```python
from build123d import *

# Parameters (mm, degrees)
SKETCH_1_R          = 1.525
SKETCH_1_R_2        = 5
EXTRUDE_1_DEPTH     = 4
CUT_EXTRUDE_START   = -4
CUT_EXTRUDE_1_DEPTH = 4
FILLET_1_R          = 1


with BuildPart() as part:
    # 草图1 → 凸台-拉伸1 (new body)
    # profile 1 of 2: a face of its own
    with BuildSketch(Plane.XY):
        with BuildLine():
            ThreePointArc((12, 0), (7.073549415, 9.693549333), (-3.660816447, 11.427966702))
            ThreePointArc((-3.660816447, 11.427966702), (-10.576904144, -5.668253587), (7.48855525, -9.376648669))
            ThreePointArc((7.48855525, -9.376648669), (10.813479158, -5.202755856), (12, 0))
        make_face()
        with Locations((5.142300877, -6.128355545)):
            Circle(SKETCH_1_R, mode=Mode.SUBTRACT)
        with Locations((-6.128355545, -5.142300877)):
            Circle(SKETCH_1_R, mode=Mode.SUBTRACT)
        Circle(SKETCH_1_R_2, mode=Mode.SUBTRACT)
        with Locations((-5.142300877, 6.128355545)):
            Circle(SKETCH_1_R, mode=Mode.SUBTRACT)
        with Locations((6.128355545, 5.142300877)):
            Circle(SKETCH_1_R, mode=Mode.SUBTRACT)
    # profile 2 of 2: a face of its own
    with BuildSketch(Plane.XY):
        with BuildLine():
            Line((25.489995997, 5), (25.489995997, 15))
            Line((25.489995997, 15), (7.489995997, 15))
            Line((7.489995997, 15), (-3.660816447, 11.427966702))
            ThreePointArc((-3.660816447, 11.427966702), (7.073549415, 9.693549333), (12, 0))
            ThreePointArc((12, 0), (10.813479158, -5.202755856), (7.48855525, -9.376648669))
            Line((7.48855525, -9.376648669), (25.489995997, 5))
        make_face()
        with Locations((12.489995997, 10)):
            Circle(SKETCH_1_R, mode=Mode.SUBTRACT)
        with Locations((20.489995997, 10)):
            Circle(SKETCH_1_R, mode=Mode.SUBTRACT)
    extrude(amount=EXTRUDE_1_DEPTH)

    # 草图2 → 切除-拉伸1 (cut)
    with BuildSketch(Plane.XY.offset(4).offset(CUT_EXTRUDE_START)):
        with BuildLine():
            ThreePointArc((12, 0), (11.855024322, -1.85967694), (11.42360028, -3.674419227))
            Line((11.42360028, -3.674419227), (18.489995997, 1.969078425))
            Line((18.489995997, 1.969078425), (18.489995997, 5))
            Line((18.489995997, 5), (10.908712115, 5))
            ThreePointArc((10.908712115, 5), (11.724004123, 2.558852734), (12, 0))
        make_face()
    extrude(amount=CUT_EXTRUDE_1_DEPTH, mode=Mode.SUBTRACT)

    # 圆角1
    fillet_1_edges = [part.edges().sort_by_distance(p)[0] for p in [
        (7.489995997, 15, 2),
        (25.489995997, 15, 2),
        (25.489995997, 5, 2),
        (11.42360028, -3.674419227, 2),
        (10.908712115, 5, 2),
        (18.489995997, 5, 2),
        (18.489995997, 1.969078425, 2),
    ]]
    fillet(fillet_1_edges, radius=FILLET_1_R)


solid = part.part
```
Work out the finished part from the listing and answer in its coordinate system (mm). A direction names the side the tool comes from. Round coordinates to 2 decimals unless told otherwise and drop trailing zeros. Write each loop counter-clockwise with the first axis right and the second up, starting at its lowest first coordinate (ties: lowest second). Pieces come first, ordered by that corner, then holes.
1) A cutting plane is placed at D-D on x = -9.5. Determine the outline of the cut face in (y, z).
2) A cutting plane is placed at C-C on z = 3.3. Give the number of separate pieces and of enclosed holes in the cut face, and give its area (3 significant figures).
3) Determine the mould class of faces 1 (the face through (25.49, 10, 2)), 2 (the face through (-4.674, -4.684, 1.972)), 3 (the face through (16.178, -2.437, 1.972)) for opening direction Y: pulls with the +Y half, pulls with the -Y half, needs draft (parallel to the pull), parting line crosses it, or undercut.
4) Which of the six approach directions +Z, -Z, +X, -X, +Y, -Y give full straight-line access (tool end or side, diameter ignored) to faces 4 (the face through (1.917, 13.215, 1.972)), 5 (the face through (18.49, 3, 2))?
5) Consider probe 1 along X at (y, z) = (9.5, 0.65); probe 2 along X at (y, z) = (-5.5, 3.1); probe 3 along Y at (x, z) = (13.5, 0.4). Determine where each line is inside the solid, lowest interval first.
6) Flat-ended cylindrical pins translate along their axes: P1, Ø1.5, axis at y = 2.5, z = 3.5, coming from the -X side; P2, Ø1.7, axis at y = 3, z = 2, coming from the -X side; P3, Ø2.5, axis at x = 6.13, y = 5.14, coming from the -Z side; P4, Ø2, axis at y = 5, z = 1, coming from the -X side. Find the tip coordinate at first contact, or state that the pin passes through.
7) A cutting plane is placed at B-B on y = 10. Determine the outline of the cut face in (x, z) (3 decimals), and give its area (3 significant figures).
8) A cutting plane is placed at A-A on x = 1. Determine the outline of the cut face in (y, z), and give its area (3 significant figures).
Entries:
1. outline: (-7.33, 0) - (7.33, 0) - (7.33, 4) - (-7.33, 4) - close
2. separate pieces: 1
2. enclosed holes: 8
2. area: 564 mm2
3. face 1: needs draft
3. face 2: undercut
3. face 3: pulls with the -Y half
4. face 4: +Z, -Z, -X, +Y
4. face 5: +Z, -Z
5. probe 1: x = -7.33 to 11.05, 13.93 to 19.05, 21.93 to 25.49
5. probe 2: x = -10.67 to -7.61, -4.65 to 3.75, 6.53 to 12.34
5. probe 3: y = -4.58 to -2.01, 5 to 8.86, 11.14 to 15
6. P1: stops at x = -11.87
6. P2: stops at x = -11.81
6. P3: passes through
6. P4: stops at x = -11.31
7. outline: (-6.633, 0) - (10.965, 0) - (10.965, 4) - (-6.633, 4) - close; (14.015, 0) - (18.965, 0) - (18.965, 4) - (14.015, 4) - close; (22.015, 0) - (25.49, 0) - (25.49, 4) - (22.015, 4) - close
7. area: 104 mm2
8. outline: (-11.96, 0) - (-4.9, 0) - (-4.9, 4) - (-11.96, 4) - close; (4.9, 0) - (12.92, 0) - (12.92, 4) - (4.9, 4) - close
8. area: 60.3 mm2
